Geometry check sheet. Reference: drawing and pictorial views, mm from the part's lowest x, y, z. Give positions to 0.01 mm unless a question says otherwise; leave off trailing zeros. Write each loop counter-clockwise with the first axis right and the second up, starting at its lowest first coordinate (ties: lowest second). Pieces come first, ordered by that corner, then holes.
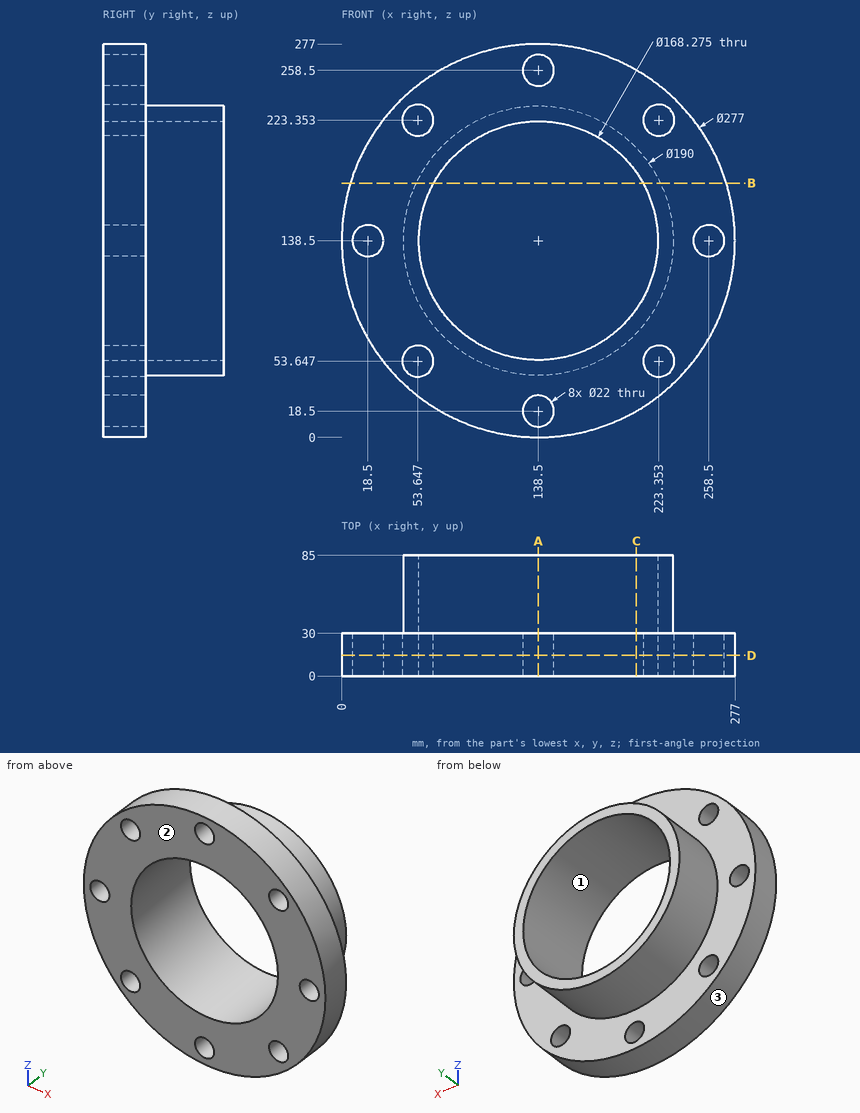
Item 1: Release check for a two-part mould opening along X. For the marked faces 1, 2 and 3 record: released by +X, released by -X, zero draft, split by the parting line, or undercut.
Answer key:
face 1: undercut
face 2: zero draft
face 3: split by the parting line
Item 2: Depth check by flat-ended pin: pin 1 (13 mm diameter, centred on x = 53.65, z = 223.35, fed in from -Y); pin 2 (2 mm diameter, centred on y = 17.5, z = 179, fed in from +X); pin 3 (1.5 mm diameter, centred on x = 92.5, y = 22.5, fed in from +Z); pin 4 (12 mm diameter, centred on x = 75.5, y = 72, fed in from +Z). Enter the tip coordinate at first touch or a pass-through.
Answer key:
pin 1: passes through
pin 2: stops at x = 271.25
pin 3: stops at z = 269.4
pin 4: stops at z = 214.5
Item 3: Sectioned sample at A-A on x = 138.5. Record the cut outline in (y, z).
Answer key:
outline: (0, 0) - (30, 0) - (30, 7.5) - (0, 7.5) - close; (0, 29.5) - (30, 29.5) - (30, 43.5) - (85, 43.5) - (85, 54.36) - (0, 54.36) - close; (0, 222.64) - (85, 222.64) - (85, 233.5) - (30, 233.5) - (30, 247.5) - (0, 247.5) - close; (0, 269.5) - (30, 269.5) - (30, 277) - (0, 277) - close
Item 4: Sectioned sample at C-C on x = 207.5. Record the cut outline in (y, z).
Answer key:
outline: (0, 18.41) - (30, 18.41) - (30, 73.2) - (85, 73.2) - (85, 90.35) - (0, 90.35) - close; (0, 186.65) - (85, 186.65) - (85, 203.8) - (30, 203.8) - (30, 258.59) - (0, 258.59) - close
Item 5: Sectioned sample at D-D on y = 14.5. State how many separate pieces and enclosed holes the cut face has, then the cut area to 3 significant figures.
Answer key:
separate pieces: 1
enclosed holes: 9
area: 35,000 mm2
Item 6: Scan lines: line 1 along Z through (x, y) = (138.5, 16.25); line 2 along X through (y, z) = (23, 138); line 3 along X through (y, z) = (23, 129) (1 decimal). Record each from-to range of solid material in increasing order.
Answer key:
line 1: z = 0 to 7.5, 29.5 to 54.36, 222.64 to 247.5, 269.5 to 277
line 2: x = 0 to 7.51, 29.49 to 54.36, 222.64 to 247.51, 269.49 to 277
line 3: x = 0.3 to 13, 24 to 54.9, 222.1 to 253, 264 to 276.7
Item 7: Sectioned sample at B-B on z = 179. Record the cut outline in (x, y).
Answer key:
outline: (6.05, 0) - (64.75, 0) - (64.75, 85) - (52.57, 85) - (52.57, 30) - (6.05, 30) - close; (212.25, 0) - (270.95, 0) - (270.95, 30) - (224.43, 30) - (224.43, 85) - (212.25, 85) - close
